from build123d import *

# Parameters (mm, degrees)
F3_R     = 32
F4_DEPTH = 5


with BuildPart() as f2:
    # F1 (on Front) → F2 (revolve)
    with BuildSketch(Plane.XZ):
        with BuildLine():
            Line((0, 43.752931), (0, 45.5))
            Line((0, 45.5), (-2.439834, 45.5))
            ThreePointArc((-2.439834, 45.5), (-2.898695, 45.355322), (-3.191588, 44.973616))
            Line((-3.191588, 44.973616), (-5.729777, 38))
            Line((-5.729777, 38), (-15.729777, 38))
            Line((-15.729777, 38), (-15.729777, 0))
            Line((-15.729777, 0), (23.5, 0))
            Line((23.5, 0), (23.5, 32))
            Line((23.5, 32), (0, 32))
            Line((0, 32), (0, 39.747069))
            ThreePointArc((0, 39.747069), (-0.132891, 40.188619), (-0.487415, 40.483473))
            Line((-0.487415, 40.483473), (-0.868877, 40.645394))
            ThreePointArc((-0.868877, 40.645394), (-1.6, 41.75), (-0.868877, 42.854606))
            Line((-0.868877, 42.854606), (-0.487415, 43.016527))
            ThreePointArc((-0.487415, 43.016527), (-0.132891, 43.311381), (0, 43.752931))
        make_face()
    revolve(axis=Axis((-0.354707, 0, 0), (1, 0, 0)))

    # F3 (on face) → F4 (cut)
    with BuildSketch(Plane.YZ.offset(23.5)):
        Circle(F3_R)
    extrude(amount=-F4_DEPTH, mode=Mode.SUBTRACT)


solid = f2.part
The model under review builds one solid part; all positions refer to its coordinate system, in mm. A direction names the side the tool comes from. Coordinates: 2 decimals unless noted, no trailing zeros. Write each loop counter-clockwise with the first axis right and the second up, starting at its lowest first coordinate (ties: lowest second). Pieces come first, ordered by that corner, then holes. Notation, with made-up numbers: (58, -20.5) - (98, -20.5) arc R23 cw to (98, 9.5) - close; hole circle Ø7 at (72.25, 16). An arc over 180 degrees is marked (long way). Answer as a JSON object with one key per item and string values. Group by question number.
1. To check wall thickness, follow probe 1 along Z at (x, y) = (15, -1); probe 2 along Z at (x, y) = (-3, -26); probe 3 along X at (y, z) = (-32, 23.5). State the ranges of each line that lie inside material, in increasing order.
2. Add section A-A (z = 0). Give the boundary of the cut face in (x, y), plus the area to 3 significant figures.
3. Clearance check with flat-ended pins moving along their axes: pin 1 Ø4 at (x, z) = (10, -24) entering from -Y; pin 2 Ø10 at (x, z) = (11.5, -34) entering from +Y; pin 3 Ø1.5 at (x, y) = (-2.5, 31.5) entering from +Z. State where each tip first meets the part, or that it passes through.
4. Add section C-C (x = 15). Give the boundary of the cut face in (y, z), plus the area to 3 significant figures.
5. Machinability: for faces 1 (the face through (18.5, 0, 0)), 2 (the face through (-10.8, 33.713, 17.535)), 3 (the face through (0, -18, 27)), which of the approach directions +Z, -Z, +X, -X, +Y, -Y give a long, thin tool a straight path to every point of the face, cutting with its end or side? Answer none if there is none.
Findings:
{
 "1": {"probe 1": "-31.98 to 31.98", "probe 2": "-37.06 to 37.06", "probe 3": "-5.11 to 0"},
 "2": {"outline": "(-15.73, -38) - (-5.73, -38) - (-3.19, -44.97) arc R0.8 ccw to (-2.44, -45.5) - (0, -45.5) - (0, -43.75) arc R0.8 ccw to (-0.49, -43.02) - (-0.87, -42.85) arc R1.2 cw to (-0.87, -40.65) - (-0.49, -40.48) arc R0.8 ccw to (0, -39.75) - (0, -32) - (18.5, -32) - (18.5, 32) - (0, 32) - (0, 39.75) arc R0.8 ccw to (-0.49, 40.48) - (-0.87, 40.65) arc R1.2 cw to (-0.87, 42.85) - (-0.49, 43.02) arc R0.8 ccw to (0, 43.75) - (0, 45.5) - (-2.44, 45.5) arc R0.8 ccw to (-3.19, 44.97) - (-5.73, 38) - (-15.73, 38) - close", "area": "2,440 mm²"},
 "3": {"pin 1": "y = -23.24", "pin 2": "y = 13.53", "pin 3": "z = 33.54"},
 "4": {"outline": "circle Ø64 at (0, 0)", "area": "3,220 mm²"},
 "5": {"face 1": "+Z, -Z, +X, +Y, -Y", "face 2": "-X", "face 3": "+X"}
}
